Geometry: final body of the model. Coordinates: model frame, mm. A direction names the side the tool comes from. Give positions to 0.01 mm unless a question says otherwise; leave off trailing zeros. Write each loop counter-clockwise with the first axis right and the second up, starting at its lowest first coordinate (ties: lowest second). Pieces come first, ordered by that corner, then holes. Notation, with made-up numbers: (73.5, 43) - (107.5, 43) arc R21 cw to (107.5, 64) - close; hole circle Ø9 at (77.5, 84.25). An arc over 180 degrees is marked (long way). Use CSV: the item, a comma, the result in double quotes. Start each with the question number.
(1) Section A-A on z = 5.5. Output: boundary loops of the cut face in (x, y), and give its area (3 significant figures).
(2) First-contact query: pin 1 Ø2.5 at (x, z) = (0, -5.5) entering from +Y; pin 2 Ø8 at (x, y) = (-5.5, 28) entering from +Z. Flat tips, straight axial feed; report the tip coordinate or a pass-through.
(3) Section B-B on y = 29.5. Output: boundary loops of the cut face in (x, z).
(4) Section D-D on z = -2.5. Output: boundary loops of the cut face in (x, y), and give its area (3 significant figures).
(5) Line query: probe 1 along X at (y, z) = (42.25, -5.5); probe 2 along Y at (x, z) = (-1.5, -1); probe 3 along Z at (x, y) = (4.75, 29). Output: solid intervals per line, ascending. Write a range as [from, to].
(6) Reachability of faces 1 (the cylindrical face through (7.07, 39.55, 0.13)), 2 (the flat face through (0, 40, 0)) from +Z, -Z, +X, -X, +Y, -Y: full face, straight path, thin tool, end or side. Return the list, or none.
(7) Draft query along Z for faces 3 (the cylindrical face through (-6.64, 20.26, 11.6)), 4 (the cylindrical face through (0.06, 0.45, -12.07)), 5 (the cylindrical face through (-0.751, 40.213, 3.115)). Return one class per face: released by +Z, released by -Z, zero draft, split by the parting line, or undercut.
from build123d import *

# Parameters (mm, degrees)
CROQUIS1_W              = 15
CROQUIS1_H              = 25
SALIENTE_EXTRUIR1_DEPTH = 40
REDONDEO1_R             = 3
REDONDEO2_R             = 1.5
REDONDEO3_R             = 1.5
CROQUIS2_R              = 2.5
SALIENTE_EXTRUIR2_DEPTH = 3
CROQUIS3_R              = 1.487403204
CORTAR_EXTRUIR1_DEPTH   = 1.5
REDONDEO4_R             = 0.5
CHAFL_N1_SIZE           = 0.2
CROQUIS4_R              = 1.299235838
CHAFL_N2_SIZE           = 0.2


with BuildPart() as part:
    # Croquis1 → Saliente-Extruir1 (new body)
    with BuildSketch(Plane(origin=(0, 0, 0), x_dir=(1, 0, 0), z_dir=(0, 1, 0))):
        Rectangle(CROQUIS1_W, CROQUIS1_H)
    extrude(amount=SALIENTE_EXTRUIR1_DEPTH)

    # Redondeo1
    redondeo1_edges = [part.edges().sort_by_distance(p)[0] for p in [
        (7.5, 20, 12.5),
        (-7.5, 20, 12.5),
        (-7.5, 20, -12.5),
        (7.5, 20, -12.5),
    ]]
    fillet(redondeo1_edges, radius=REDONDEO1_R)

    # Redondeo2
    redondeo2_edges = [part.edges().sort_by_distance(p)[0] for p in [
        (-7.5, 0, 0),
        (7.5, 0, 0),
        (0, 0, 12.5),
        (0, 0, -12.5),
        (6.621320344, 0, 11.621320344),
        (-6.621320344, 0, 11.621320344),
        (6.621320344, 0, -11.621320344),
        (-6.621320344, 0, -11.621320344),
    ]]
    fillet(redondeo2_edges, radius=REDONDEO2_R)

    # Redondeo3
    redondeo3_edges = [part.edges().sort_by_distance(p)[0] for p in [
        (-7.5, 40, 0),
        (0, 40, -12.5),
        (7.5, 40, 0),
        (0, 40, 12.5),
        (6.621320344, 40, 11.621320344),
        (-6.621320344, 40, 11.621320344),
        (6.621320344, 40, -11.621320344),
        (-6.621320344, 40, -11.621320344),
    ]]
    fillet(redondeo3_edges, radius=REDONDEO3_R)

    # Croquis2 → Saliente-Extruir2 (add)
    with BuildSketch(Plane(origin=(0, 40, 0), x_dir=(1, 0, 0), z_dir=(0, 1, 0))):
        with Locations(Location((0, 5.5, 0), (0, 0, 270))):
            Circle(CROQUIS2_R)
        with Locations(Location((0, -5.5, 0), (0, 0, 90))):
            Circle(CROQUIS2_R)
    extrude(amount=SALIENTE_EXTRUIR2_DEPTH)

    # Croquis3 → Cortar-Extruir1 (cut)
    with BuildSketch(Plane(origin=(0, 43, 0), x_dir=(1, 0, 0), z_dir=(0, 1, 0))):
        with Locations(Location((0, 5.5, 0), (0, 0, 270))):
            Circle(CROQUIS3_R)
    extrude(amount=-CORTAR_EXTRUIR1_DEPTH, mode=Mode.SUBTRACT)

    # Redondeo4
    redondeo4_edges = [part.edges().sort_by_distance(p)[0] for p in [
        (0, 43, -6.987403204),
    ]]
    fillet(redondeo4_edges, radius=REDONDEO4_R)

    # Chaflán1
    chafl_n1_edges = [part.edges().sort_by_distance(p)[0] for p in [
        (0, 43, -8),
    ]]
    chamfer(chafl_n1_edges, length=CHAFL_N1_SIZE)

    # Croquis4 → Cortar-Revolución1 (revolve, cut)
    with BuildSketch(Plane(origin=(0, 0, 0), x_dir=(0, 0, -1), z_dir=(1, 0, 0))):
        with Locations((-2.260920396, 41.5)):
            Circle(CROQUIS4_R)
    revolve(axis=Axis((0, 43, 5.5), (0, -1, 0)), mode=Mode.SUBTRACT)

    # Chaflán2
    chafl_n2_edges = [part.edges().sort_by_distance(p)[0] for p in [
        (0, 43, 8),
    ]]
    chamfer(chafl_n2_edges, length=CHAFL_N2_SIZE)


solid = part.part
Check values:
1,outline,"(-7.5, 1.5) arc R1.5 ccw to (-6, 0) - (6, 0) arc R1.5 ccw to (7.5, 1.5) - (7.5, 38.5) arc R1.5 ccw to (6, 40) - (2.5, 40) - (2.5, 40.43) arc R1.3 cw to (2.5, 42.57) - (2.5, 42.8) - (2.3, 43) - (-2.3, 43) - (-2.5, 42.8) - (-2.5, 42.57) arc R1.3 cw to (-2.5, 40.43) - (-2.5, 40) - (-6, 40) arc R1.5 ccw to (-7.5, 38.5) - close"
1,area,"611 mm²"
2,pin 1,"stops at y = 41.5"
2,pin 2,"stops at z = 12.5"
3,outline,"(-7.5, -9.5) arc R3 ccw to (-4.5, -12.5) - (4.5, -12.5) arc R3 ccw to (7.5, -9.5) - (7.5, 9.5) arc R3 ccw to (4.5, 12.5) - (-4.5, 12.5) arc R3 ccw to (-7.5, 9.5) - close"
4,outline,"(-7.5, 1.5) arc R1.5 ccw to (-6, 0) - (6, 0) arc R1.5 ccw to (7.5, 1.5) - (7.5, 38.5) arc R1.5 ccw to (6, 40) - (-6, 40) arc R1.5 ccw to (-7.5, 38.5) - close"
4,area,"598 mm²"
5,probe 1,"x = [-2.5, -1.49], [1.49, 2.5]"
5,probe 2,"y = [0, 40]"
5,probe 3,"z = [-12.49, 12.49]"
6,face 1,"+Z, -Z, +X, +Y"
6,face 2,"+Y"
7,face 3,"released by +Z"
7,face 4,"released by -Z"
7,face 5,"undercut"
